from build123d import *

# Parameters (mm, degrees)
SALIENTE_EXTRUIR1_DEPTH = 3
CROQUIS2_R              = 2.8
CORTAR_EXTRUIR1_DEPTH   = 10
CROQUIS3_R              = 5
CORTAR_EXTRUIR2_DEPTH   = 10
REDONDEO1_R             = 10


with BuildPart() as part:
    # Croquis1 → Saliente-Extruir1 (new body)
    with BuildSketch(Plane.XY):
        with BuildLine():
            Line((-13.118348224, -13.346885602), (-5.358962429, -8.729934305))
            ThreePointArc((-5.358962429, -8.729934305), (0, -10.243545836), (5.358962429, -8.729934305))
            Line((5.358962429, -8.729934305), (13.118348224, -13.346885602))
            ThreePointArc((13.118348224, -13.346885602), (19.97194541, -11.606711584), (18.231771393, -4.753114398))
            Line((18.231771393, -4.753114398), (10.243545836, 0))
            ThreePointArc((10.243545836, 0), (8.83594818, 5.182301714), (5, 8.94037087))
            Line((5, 8.94037087), (5, 18.2))
            ThreePointArc((5, 18.2), (0, 23.2), (-5, 18.2))
            Line((-5, 18.2), (-5, 8.94037087))
            ThreePointArc((-5, 8.94037087), (-8.83594818, 5.182301714), (-10.243545836, 0))
            Line((-10.243545836, 0), (-18.231771393, -4.753114398))
            ThreePointArc((-18.231771393, -4.753114398), (-19.97194541, -11.606711584), (-13.118348224, -13.346885602))
        make_face()
    extrude(amount=SALIENTE_EXTRUIR1_DEPTH)

    # Croquis2 → Cortar-Extruir1 (cut)
    with BuildSketch(Plane.XY.offset(3)):
        with Locations((0, 18.2)):
            Circle(CROQUIS2_R)
        with Locations((15.675059808, -9.05)):
            Circle(CROQUIS2_R)
        with Locations((-15.675059808, -9.05)):
            Circle(CROQUIS2_R)
    extrude(amount=-CORTAR_EXTRUIR1_DEPTH, mode=Mode.SUBTRACT)

    # Croquis3 → Cortar-Extruir2 (cut)
    with BuildSketch(Plane.XY.offset(3)):
        Circle(CROQUIS3_R)
    extrude(amount=-CORTAR_EXTRUIR2_DEPTH, mode=Mode.SUBTRACT)

    # Redondeo1
    redondeo1_edges = [part.edges().sort_by_distance(p)[0] for p in [
        (-10.243545836, 0, 1.5),
        (-5, 8.94037087, 1.5),
        (5, 8.94037087, 1.5),
        (10.243545836, 0, 1.5),
        (5.358962429, -8.729934305, 1.5),
        (-5.358962429, -8.729934305, 1.5),
    ]]
    fillet(redondeo1_edges, radius=REDONDEO1_R)


solid = part.part
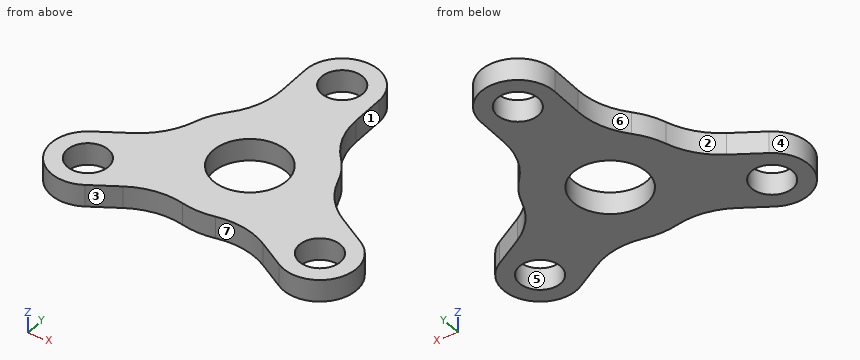
Work out the finished part from the listing and answer in its coordinate system (mm). Face numbers are marked on the shaded views. A direction names the side the tool comes from. Round coordinates to 2 decimals unless told otherwise and drop trailing zeros. Loops run counter-clockwise (first coordinate to the right, second up) from the corner with the lowest first, then second, coordinate; pieces in that order, holes last. Notation, with made-up numbers: (-34, 4) - (8, 4) arc R29 cw to (8, 30) - close; hole circle Ø6 at (23.5, -9.5). An arc over 180 degrees is marked (long way). Use one line per item in the form item = value. Start each with the question number.
(1) Flat-ended cylindrical pins translate along their axes: P1, Ø1.5, axis at x = 1.5, z = 1.5, coming from the +Y side; P2, Ø1, axis at x = 0, z = 1.5, coming from the -Y side; P3, Ø1.5, axis at y = 16, z = 1.5, coming from the +X side; P4, Ø5, axis at x = -15.68, y = -9.05, coming from the +Z side. Find the tip coordinate at first contact, or state that the pin passes through.
(2) Find section D-D on y = -3.5. Determine the outline of the cut face in (x, z).
(3) Find section B-B on z = 2.25. Determine the outline of the cut face in (x, y), and give its area (3 significant figures).
(4) Consider line 1 (Y direction, x = 0, z = 1.7); line 2 (X direction, y = -12, z = 1.15); line 3 (Y direction, x = -3, z = 0.55). Determine where each line is inside the solid, lowest interval first.
(5) Find section A-A on y = -9.05. Determine the outline of the cut face in (x, z), and give its area (3 significant figures).
(6) Find section C-C on x = 0. Determine the outline of the cut face in (y, z), and give its area (3 significant figures).
(7) Which of the six approach directions +Z, -Z, +X, -X, +Y, -Y give full straight-line access (tool end or side, diameter ignored) to the marked faces 1, 2 and 3?
(8) Determine the mould class of the marked faces 4, 5, 6 and 7 for opening direction Y: +Y half, -Y half, draft (parallel to the pull), parting line (faces both ways), or undercut.
Answer list:
q1.P1 = 23.14
q1.P2 = -10.24
q1.P3 = 5
q1.P4 = through
q2.outline = (-16.13, 0) - (-3.57, 0) - (-3.57, 3) - (-16.13, 3) - close; (3.57, 0) - (16.13, 0) - (16.13, 3) - (3.57, 3) - close
q3.outline = (-18.23, -4.75) arc R5 ccw to (-13.12, -13.35) - (-9.47, -11.18) arc R10 cw to (-2.2, -10) arc R10.24 ccw to (2.2, -10) arc R10 cw to (9.47, -11.18) - (13.12, -13.35) arc R5 ccw to (18.23, -4.75) - (14.13, -2.31) arc R10 cw to (9.74, 3.18) arc R10.24 ccw to (7.59, 6.88) arc R10 cw to (5, 13.59) - (5, 18.2) arc R5 ccw to (-5, 18.2) - (-5, 13.59) arc R10 cw to (-7.59, 6.88) arc R10.24 ccw to (-9.74, 3.18) arc R10 cw to (-14.13, -2.31) - close; hole circle Ø5.6 at (-15.68, -9.05); hole circle Ø10 at (0, 0); hole circle Ø5.6 at (0, 18.2); hole circle Ø5.6 at (15.68, -9.05)
q3.area = 559 mm^2
q4.line_1 = -10.24 to -5, 5 to 15.4, 21 to 23.2
q4.line_2 = -19.71 to -10.85, 10.85 to 19.71
q4.line_3 = -9.86 to -4, 4 to 22.2
q5.outline = (-20.68, 0) - (-18.48, 0) - (-18.48, 3) - (-20.68, 3) - close; (-12.88, 0) - (12.88, 0) - (12.88, 3) - (-12.88, 3) - close; (18.48, 0) - (20.68, 0) - (20.68, 3) - (18.48, 3) - close
q5.area = 90.5 mm^2
q6.outline = (-10.24, 0) - (-5, 0) - (-5, 3) - (-10.24, 3) - close; (5, 0) - (15.4, 0) - (15.4, 3) - (5, 3) - close; (21, 0) - (23.2, 0) - (23.2, 3) - (21, 3) - close
q6.area = 53.5 mm^2
q7.face_1 = +Z, -Z, +X, +Y
q7.face_2 = +Z, -Z, -X, +Y
q7.face_3 = +Z, -Z, -Y
q8.face_4 = parting line
q8.face_5 = undercut
q8.face_6 = +Y half
q8.face_7 = -Y half
